```python
from build123d import *

# Parameters (mm, degrees)
SKETCH1_W                    = 76.2
SKETCH1_H                    = 25.4
BASE_FLANGE1_DEPTH           = 0.7366
EDGE_FLANGE1_STRIP_W         = 4.4196
EDGE_FLANGE1_STRIP_H         = 0.7366
EDGE_FLANGE1_STRIP_CUT_DEPTH = 76.2
EDGE_FLANGE1_DEPTH           = 76.2


# Sheet-metal steps are written as plain solids
with BuildPart() as part:
    # Sketch1 → Base-Flange1 (new body)
    with BuildSketch(Plane(origin=(0, 0, 0), x_dir=(1, 0, 0), z_dir=(0, 1, 0))):
        with Locations((38.1, 12.7)):
            Rectangle(SKETCH1_W, SKETCH1_H)
    extrude(amount=-BASE_FLANGE1_DEPTH)

    # Edge-Flange1 strip (across the edge) → Edge-Flange1 strip cut (cut)
    with BuildSketch(Plane(origin=(76.2, 0, -25.4), x_dir=(0, 0, 1), z_dir=(-1, 0, 0))):
        with Locations((-1.4732, -0.3683)):
            Rectangle(EDGE_FLANGE1_STRIP_W, EDGE_FLANGE1_STRIP_H)
    extrude(amount=EDGE_FLANGE1_STRIP_CUT_DEPTH, mode=Mode.SUBTRACT)

    # Edge-Flange1 section (across the edge) → Edge-Flange1 (add)
    with BuildSketch(Plane(origin=(76.2, 0, -25.4), x_dir=(0, 0, 1), z_dir=(-1, 0, 0))):
        with BuildLine():
            Line((-0.7366, 0.7366), (-0.7366, 111.76))
            Line((-0.7366, 111.76), (0, 111.76))
            Line((0, 111.76), (0, 0.7366))
            ThreePointArc((0, 0.7366), (0.215745145, 0.215745145), (0.7366, 0))
            Line((0.7366, 0), (0.7366, -0.7366))
            ThreePointArc((0.7366, -0.7366), (-0.30510971, -0.30510971), (-0.7366, 0.7366))
        make_face()
    extrude(amount=EDGE_FLANGE1_DEPTH)


solid = part.part
```
Can you work these out from the model? Positions are in its coordinate system, mm. A direction names the side the tool comes from. Give positions to 0.01 mm unless a question says otherwise; leave off trailing zeros. Write each loop counter-clockwise with the first axis right and the second up, starting at its lowest first coordinate (ties: lowest second). Pieces come first, ordered by that corner, then holes. Notation, with made-up numbers: (87, 38.25) - (104, 38.25) arc R23 ccw to (104, 55.25) - close; hole circle Ø1 at (-19.75, 58.25). An arc over 180 degrees is marked (long way). Write item = value, one per line. Start each with the question number.
1. For pin 1 (10 mm diameter, centred on x = 65.5, y = 77, fed in from +Z); pin 2 (12.5 mm diameter, centred on x = 32, z = -6, fed in from +Y), each with a flat end and sliding along its axis, tell me the tip position at first contact or that it passes through.
2. Imagine slicing it at B-B (y = 80.5). Please give me the cut outline in (x, z), and give its area (3 significant figures).
3. Imagine slicing it at C-C (z = -5.75). Please give me the cut outline in (x, y).
4. Imagine slicing it at A-A (x = 31.5). Please give me the cut outline in (y, z).
5. Please list where these lines run through material, in increasing order: line 1 (Y direction, x = 23, z = -8.5); line 2 (Z direction, x = 53.5, y = 70).
6. On a 3-axis mill with a long thin cutter (end or side, diameter ignored), from which of +Z, -Z, +X, -X, +Y, -Y can I reach the whole of each face in a straight line? I mean faces 1 (the face through (39, 55, -26.137)), 2 (the face through (39, 57, -25.4)). Say none if no direction works.
Worked answers:
q1.pin_1 = -25.4
q1.pin_2 = 0
q2.outline = (0, -26.14) - (76.2, -26.14) - (76.2, -25.4) - (0, -25.4) - close
q2.area = 56.1 mm2
q3.outline = (0, -0.74) - (76.2, -0.74) - (76.2, 0) - (0, 0) - close
q4.outline = (-0.74, -24.66) arc R1.47 ccw to (0.74, -26.14) - (111.76, -26.14) - (111.76, -25.4) - (0.74, -25.4) arc R0.74 cw to (0, -24.66) - (0, 0) - (-0.74, 0) - close
q5.line_1 = -0.74 to 0
q5.line_2 = -26.14 to -25.4
q6.face_1 = -Z, +X, -X, +Y, -Y
q6.face_2 = +Z, +X, -X, +Y
